Answer from the drawing. Dimensions are ordinates in mm from the lowest x, y and z of the part. Round coordinates to 2 decimals unless told otherwise and drop trailing zeros. Write each loop counter-clockwise with the first axis right and the second up, starting at its lowest first coordinate (ties: lowest second). Pieces come first, ordered by that corner, then holes. Notation, with made-up numbers: M -9.75,44 L -0.75,44 A15 cw -0.75,49 Z; hole C -9.5,-19.5 d6. An arc over 180 degrees is marked long. One line per item, written item: value. Start each with the question number.
(1) Section C-C (z = 1.45) is taken. Determine the outline of the cut face in (x, y).
(2) Section A-A (y = 48) is taken. Determine the outline of the cut face in (x, z), plus the area to 3 significant figures.
(3) Consider probe 1 along Y at (x, z) = (22, 1.8); probe 2 along Y at (x, z) = (22.5, 1.2); probe 3 along X at (y, z) = (25.5, 0.9). Determine where each line is inside the solid, lowest interval first.
(4) Section B-B (x = 52) is taken. Determine the outline of the cut face in (y, z), plus the area to 3 significant figures.
(5) Given P1, Ø1, axis at y = 30.5, z = 2, coming from the +X side, flat-ended and moving along its own axis, determine where the tip first touches the part or whether it passes through.
(6) Section D-D (y = 13.5) is taken. Determine the outline of the cut face in (x, z).
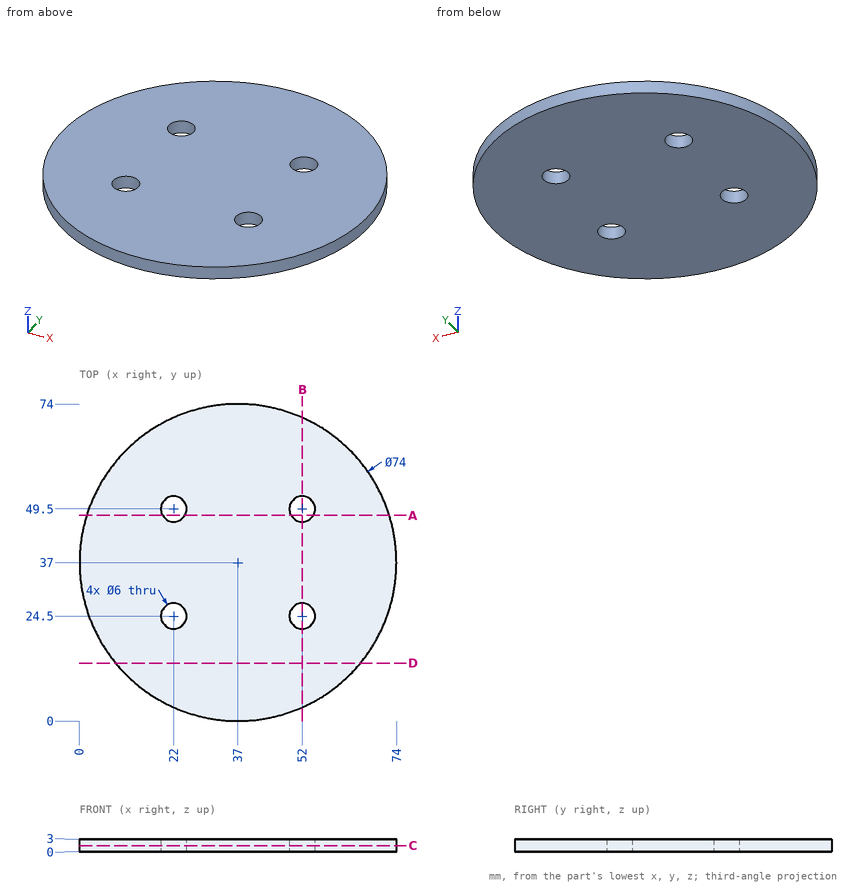
Recorded:
1. outline: C 37,37 d74; hole C 22,24.5 d6; hole C 22,49.5 d6; hole C 52,24.5 d6; hole C 52,49.5 d6
2. outline: M 1.67,0 L 19.4,0 L 19.4,3 L 1.67,3 Z; M 24.6,0 L 49.4,0 L 49.4,3 L 24.6,3 Z; M 54.6,0 L 72.33,0 L 72.33,3 L 54.6,3 Z
2. area: 181 mm2
3. probe 1: y = 3.18 to 21.5, 27.5 to 46.5, 52.5 to 70.82
3. probe 2: y = 2.96 to 21.54, 27.46 to 46.54, 52.46 to 71.04
3. probe 3: x = 1.83 to 19.17, 24.83 to 49.17, 54.83 to 72.17
4. outline: M 3.18,0 L 21.5,0 L 21.5,3 L 3.18,3 Z; M 27.5,0 L 46.5,0 L 46.5,3 L 27.5,3 Z; M 52.5,0 L 70.82,0 L 70.82,3 L 52.5,3 Z
4. area: 167 mm2
5. P1: stops at x = 73.51
6. outline: M 8.42,0 L 65.58,0 L 65.58,3 L 8.42,3 Z
